The listing builds one solid part. Answer for the finished solid, in the listing's coordinates (mm). Face numbers are marked on the shaded views. A direction names the side the tool comes from. Give positions to 0.01 mm unless a question says otherwise; leave off trailing zeros. Loops run counter-clockwise (first coordinate to the right, second up) from the corner with the lowest first, then second, coordinate; pieces in that order, holes last. Notation, with made-up numbers: (-10, -20.75) - (30, -20.75) arc R12 cw to (30, -2.75) - close; hole circle Ø8 at (-15, 62.25). An arc over 180 degrees is marked (long way). Write each question's results on one line, items separated by ' | '.
from build123d import *

# Parameters (mm, degrees)
SKETCH1_W           = 6.35
SKETCH1_H           = 49.4538
BOSS_EXTRUDE1_DEPTH = 3.175
SKETCH2_R           = 1.524
BOSS_EXTRUDE2_DEPTH = 8.89
FILLET1_R           = 3.175


with BuildPart() as part:
    # Sketch1 → Boss-Extrude1 (new body)
    with BuildSketch(Plane(origin=(0, 0, 0), x_dir=(0, 0, -1), z_dir=(1, 0, 0))):
        Rectangle(SKETCH1_W, SKETCH1_H)
    extrude(amount=BOSS_EXTRUDE1_DEPTH)

    # Sketch2 → Boss-Extrude2 (add)
    with BuildSketch(Plane.ZY):
        with Locations(Location((0, 21.5519, 0), (0, 0, 180))):
            Circle(SKETCH2_R)
        with Locations(Location((0, -21.5519, 0), (0, 0, 180))):
            Circle(SKETCH2_R)
    extrude(amount=BOSS_EXTRUDE2_DEPTH)

    # Fillet1
    fillet1_edges = [part.edges().sort_by_distance(p)[0] for p in [
        (1.5875, -24.7269, 3.175),
        (1.5875, -24.7269, -3.175),
        (1.5875, 24.7269, -3.175),
        (1.5875, 24.7269, 3.175),
    ]]
    fillet(fillet1_edges, radius=FILLET1_R - 0.0001)  # a hair under: the kernel refuses the full size


solid = part.part
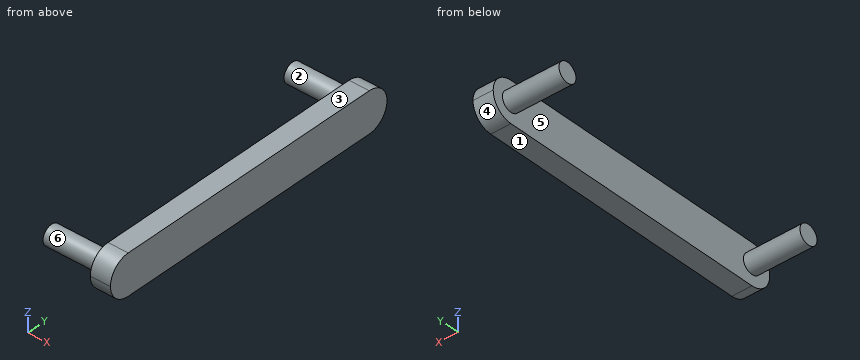
Item 1: A cutting plane is placed at A-A, the plane y = 4. Determine the outline of the cut face in (x, z) (3 decimals), plus the area to 3 significant figures.
Values found:
outline: (0, -3.175) - (3.175, -3.175) - (3.175, 3.175) - (0, 3.175) - close | area: 20.2 mm²
Item 2: A cutting plane is placed at B-B, the plane x = -1.5. Determine the outline of the cut face in (y, z), plus the area to 3 significant figures.
Values found:
outline: circle Ø3.05 at (-21.55, 0); circle Ø3.05 at (21.55, 0) | area: 14.6 mm²
Item 3: A cutting plane is placed at D-D, the plane y = 20.5. Determine the outline of the cut face in (x, z) (3 decimals), plus the area to 3 significant figures.
Values found:
outline: (-8.89, -1.103) - (0, -1.103) - (0, -3.175) - (3.175, -3.175) - (3.175, 3.175) - (0, 3.175) - (0, 1.103) - (-8.89, 1.103) - close | area: 39.8 mm²
Item 4: A flat-ended cylindrical pin translates along its axis: P1, Ø1.9, axis at y = -6.5, z = 0, coming from the -X side. Find the tip coordinate at first contact, or state that the pin passes through.
Values found:
P1: stops at x = 0
Item 5: For the marked faces 1 and 2, determine the directions among +Z, -Z, +X, -X, +Y, -Y from which every point of the face is accessible in a straight line to the end or side of a thin tool.
Values found:
face 1: -Z, +X, -X, +Y, -Y | face 2: -X
Item 6: Find the intervals of material crossed by line 1 along X through (y, z) = (17.5, -1.5) (3 decimals); line 2 along Y through (x, z) = (-5.75, 0); line 3 along Y through (x, z) = (-6.25, 0.5), in increasing order. Write a range as [from, to].
Values found:
line 1: x = [0, 3.175] | line 2: y = [-23.08, -20.03], [20.03, 23.08] | line 3: y = [-22.99, -20.11], [20.11, 22.99]
Item 7: For a pull along Y with two mould halves and no side action, classify the marked faces 3, 4, 5 and 6 as released by +Y, released by -Y, zero draft, split by the parting line, or undercut.
Values found:
face 3: zero draft | face 4: released by +Y | face 5: undercut | face 6: undercut
Item 8: A cutting plane is placed at C-C, the plane z = -0.5. Determine the outline of the cut face in (x, y) (3 decimals).
Values found:
outline: (-8.89, -22.992) - (0, -22.992) - (0, -24.687) - (3.175, -24.687) - (3.175, 24.687) - (0, 24.687) - (0, 22.992) - (-8.89, 22.992) - (-8.89, 20.112) - (0, 20.112) - (0, -20.112) - (-8.89, -20.112) - close
